Here's how the part is built. I have some questions about the finished solid (model axes, mm). Face numbers are marked on the shaded views. A direction names the side the tool comes from. Coordinates: 2 decimals unless noted, no trailing zeros. Loops run counter-clockwise (first coordinate to the right, second up) from the corner with the lowest first, then second, coordinate; pieces in that order, holes last. Notation, with made-up numbers: M 5,-21 L 10,-21 A30 ccw 10,11 Z; hole C 85.5,55 d1. An arc over 180 degrees is marked long. Use CSV: the item, a comma, the result in double quotes. Start each with the question number.
Q1. Please list where these lines run through material, in increasing order: probe 1 along Z at (x, y) = (-3.5, 0); probe 2 along X at (y, z) = (27, -21.5); probe 3 along Y at (x, z) = (-2.75, -15). Write a range as [from, to].
Q2. If we section it at C-C (x = -8.5): Please give me the cut outline in (y, z).
Q3. If we section it at A-A (y = 0): State how many separate pieces and enclosed holes the cut face has, and give its area (3 significant figures).
Q4. For pin 1 Ø9 at (y, z) = (0, -50) entering from -X; pin 2 Ø5 at (x, y) = (4, 43) entering from -Z; pin 3 Ø4 at (y, z) = (50, 0) entering from +X; pin 4 Ø1.5 at (x, y) = (1.5, 19.5) entering from -Z, each with a flat end and sliding along its axis, tell me the tip position at first contact or that it passes through.
Q5. Which directions (+Z, -Z, +X, -X, +Y, -Y) give clear straight access to the entire face, cutting with the end or side of a thin tool? Please do the marked faces 1, 2 and 3.
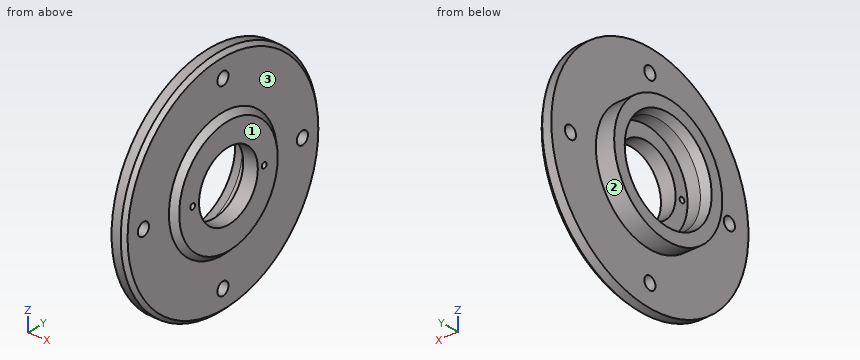
from build123d import *

# Parameters (mm, degrees)
ZKOSEN_1_SIZE            = 2
SKICA2_R                 = 1.5
ODEBRAT_VYSUNUT_M1_DEPTH = 8
KRUHOV_POLE1_COUNT       = 2
SKICA3_R                 = 3.5
ODEBRAT_VYSUNUT_M2_DEPTH = 7
KRUHOV_POLE2_COUNT       = 4


with BuildPart() as part:
    # Skica1 → Rotovat1 (revolve)
    with BuildSketch(Plane.XY):
        Polygon((-2, 62), (-2, 34), (-12, 34), (-12, 27.339745962), (-7, 26), (0, 26), (0, 18.5), (8, 18.5), (8, 31), (5, 34), (5, 62), align=None)
    revolve(axis=Axis((-20.777479893, 0, 0), (1, 0, 0)))

    # Zkosení1
    zkosen_1_edges = [part.edges().sort_by_distance(p)[0] for p in [
        (5, -62, 0),
    ]]
    chamfer(zkosen_1_edges, length=ZKOSEN_1_SIZE)

    # Skica2 → Odebrat vysunutím1 (cut)
    with BuildSketch(Plane(origin=(8, 0, 0), x_dir=(0, 0, -1), z_dir=(1, 0, 0))):
        with Locations((0, 22.5)):
            Circle(SKICA2_R)
    odebrat_vysunut_m1 = extrude(amount=-ODEBRAT_VYSUNUT_M1_DEPTH, mode=Mode.SUBTRACT)

    # Kruhové pole1: Odebrat vysunutím1 ×2 about axis
    kruhov_pole1_axis = Axis((0, 0, 0), (1, 0, 0))
    for i in range(1, KRUHOV_POLE1_COUNT):
        add(odebrat_vysunut_m1.rotate(kruhov_pole1_axis, i * 360 / KRUHOV_POLE1_COUNT), mode=Mode.SUBTRACT)

    # Skica3 → Odebrat vysunutím2 (cut)
    with BuildSketch(Plane(origin=(5, 0, 0), x_dir=(0, 0, -1), z_dir=(1, 0, 0))):
        with Locations((0, 50)):
            Circle(SKICA3_R)
    odebrat_vysunut_m2 = extrude(amount=-ODEBRAT_VYSUNUT_M2_DEPTH, mode=Mode.SUBTRACT)

    # Kruhové pole2: Odebrat vysunutím2 ×4 about axis
    kruhov_pole2_axis = Axis((0, 0, 0), (1, 0, 0))
    for i in range(1, KRUHOV_POLE2_COUNT):
        add(odebrat_vysunut_m2.rotate(kruhov_pole2_axis, i * 360 / KRUHOV_POLE2_COUNT), mode=Mode.SUBTRACT)


solid = part.part
Results below:
1,probe 1,"[-34, -26], [26, 34]"
1,probe 2,"[-2, 5]"
1,probe 3,"[-30.51, -21.24], [21.24, 30.51]"
2,outline,"C 0,0 d68; hole C 0,0 d52.8"
3,separate pieces,"4"
3,enclosed holes,"0"
3,area,"714 mm^2"
4,pin 1,"x = -2"
4,pin 2,"z = -46.76"
4,pin 3,"through"
4,pin 4,"z = -59.1"
5,face 1,"+Z, -Z, +X, +Y, -Y"
5,face 2,"-X"
5,face 3,"+X"
